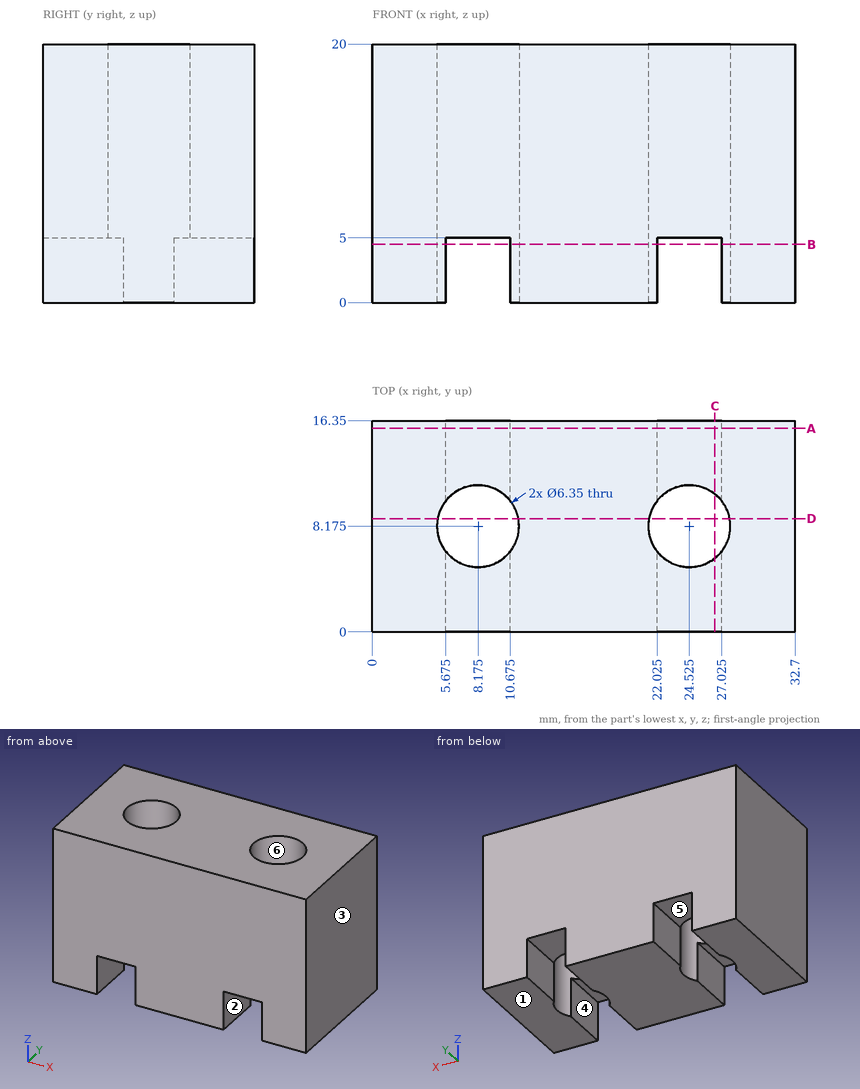
Job drawing, mm, ordinate dimensions from the low corner. One solid piece. A direction names the side the tool comes from. Give positions to 0.01 mm unless a question says otherwise; leave off trailing zeros. Write each loop counter-clockwise with the first axis right and the second up, starting at its lowest first coordinate (ties: lowest second). Pieces come first, ordered by that corner, then holes. Notation, with made-up numbers: (67, 33) -> (98, 33) arc R25 ccw to (98, 55) -> close; hole circle Ø6 at (24.5, 74). An arc over 180 degrees is marked (long way). Return JSON: item names as keys, results as strings.
Item 1: Drill centre lines: probe 1 along X at (y, z) = (10.75, 4) (3 decimals); probe 2 along X at (y, z) = (7.5, 12); probe 3 along Z at (x, y) = (9, 3.75). Where is each one in solid material? Low to high.
Answer below:
{"probe 1": "x = 0 to 5.675, 10.675 to 22.025, 27.025 to 32.7", "probe 2": "x = 0 to 5.07, 11.28 to 21.42, 27.63 to 32.7", "probe 3": "z = 5 to 20"}
Item 2: Two-plate mould, pull along X, no slides. Class the marked faces 1, 2, 3 and 4: +X half, -X half, draft (parallel to the pull), parting line (faces both ways), or undercut.
Answer below:
{"face 1": "draft", "face 2": "undercut", "face 3": "+X half", "face 4": "undercut"}
Item 3: Band-saw the part on B-B (z = 4.5). List the corners of the cut face in (x, y) (3 decimals).
Answer below:
{"outline": "(0, 0) -> (5.675, 0) -> (5.675, 6.218) arc R3.175 cw to (5.675, 10.132) -> (5.675, 16.35) -> (0, 16.35) -> close; (10.675, 0) -> (22.025, 0) -> (22.025, 6.218) arc R3.175 cw to (22.025, 10.132) -> (22.025, 16.35) -> (10.675, 16.35) -> (10.675, 10.132) arc R3.175 cw to (10.675, 6.218) -> close; (27.025, 0) -> (32.7, 0) -> (32.7, 16.35) -> (27.025, 16.35) -> (27.025, 10.132) arc R3.175 cw to (27.025, 6.218) -> close"}
Item 4: Band-saw the part on A-A (y = 15.75). List the corners of the cut face in (x, z) (3 decimals).
Answer below:
{"outline": "(0, 0) -> (5.675, 0) -> (5.675, 5) -> (10.675, 5) -> (10.675, 0) -> (22.025, 0) -> (22.025, 5) -> (27.025, 5) -> (27.025, 0) -> (32.7, 0) -> (32.7, 20) -> (0, 20) -> close"}
Item 5: Drop a flat-ended pin along its axis: pin 1 (4 mm diameter, centred on x = 24.525, y = 8.175, fed in from -Z). Give the stop position or say it passes through.
Answer below:
{"pin 1": "passes through"}
Item 6: Band-saw the part on D-D (y = 8.75). List the corners of the cut face in (x, z).
Answer below:
{"outline": "(0, 0) -> (5.05, 0) -> (5.05, 20) -> (0, 20) -> close; (11.3, 0) -> (21.4, 0) -> (21.4, 20) -> (11.3, 20) -> close; (27.65, 0) -> (32.7, 0) -> (32.7, 20) -> (27.65, 20) -> close"}
Item 7: Band-saw the part on C-C (x = 26.5). List the corners of the cut face in (y, z), then the cut area to 3 significant figures.
Answer below:
{"outline": "(0, 5) -> (5.69, 5) -> (5.69, 20) -> (0, 20) -> close; (10.66, 5) -> (16.35, 5) -> (16.35, 20) -> (10.66, 20) -> close", "area": "171 mm2"}
Item 8: Tool access for the marked faces 5 and 6: list every direction of +Z, -Z, +X, -X, +Y, -Y with a clear straight run to the whole face (end or side of a thin tool).
Answer below:
{"face 5": "-Z, +Y, -Y", "face 6": "+Z, -Z"}
